```python
from build123d import *

# Parameters (mm, degrees)
SKETCH045_W     = 10
SKETCH045_H     = 80
PAD018_DEPTH    = 7
SKETCH046_R     = 1.4
POCKET026_DEPTH = 8
SKETCH047_R     = 3.5
POCKET027_DEPTH = 80.001


with BuildPart() as part:
    # Sketch045 → Pad018 (new body)
    with BuildSketch(Plane.XY):
        with Locations((100, 0)):
            Rectangle(SKETCH045_W, SKETCH045_H)
    extrude(amount=PAD018_DEPTH)

    # Sketch046 (on Face5 of Pad018) → Pocket026 (cut)
    with BuildSketch(Plane(origin=(0, 0, 0), x_dir=(1, 0, 0), z_dir=(0, 0, -1))):
        with Locations((100, 30)):
            Circle(SKETCH046_R)
        with Locations((100, -30)):
            Circle(SKETCH046_R)
    extrude(amount=-POCKET026_DEPTH, mode=Mode.SUBTRACT)

    # Sketch047 (on Face6 of Pocket026) → Pocket027 (cut, through all)
    with BuildSketch(Plane.XZ.offset(40)):
        with Locations((107.358391, 3.5)):
            Circle(SKETCH047_R)
        with Locations((92.471756, 3.5)):
            Circle(SKETCH047_R)
    extrude(amount=-POCKET027_DEPTH, mode=Mode.SUBTRACT)


with BuildPart() as part_1:
    # Body006 placement: moved
    add(part.part.moved(Location((0, 0, 36.5))))


solid = part_1.part
```
Here's how the part is built. I have some questions about the finished solid (model axes, mm). Round coordinates to 2 decimals unless told otherwise and drop trailing zeros. Order: outer loops, then holes, each group sorted by start corner. A loop starts at its lowest first (then second) coordinate and runs counter-clockwise, first axis right, second up. Notation, with made-up numbers: M 26,83 L 39,83 A8 cw 39,93 Z; hole C 45,57 d3. An arc over 180 degrees is marked long. One line per question, with ' | ' between items.
1) For pin 1 Ø3 at (y, z) = (-24.5, 40.5) entering from -X, with a flat end and sliding along its axis, tell me the tip position at first contact or that it passes through.
Working result:
pin 1: x = 95.34
2) I want a section at B-B, the plane x = 100. Write out the boundary of the cut face in (y, z).
Working result:
outline: M -40,36.5 L -31.4,36.5 L -31.4,43.5 L -40,43.5 Z; M -28.6,36.5 L 28.6,36.5 L 28.6,43.5 L -28.6,43.5 Z; M 31.4,36.5 L 40,36.5 L 40,43.5 L 31.4,43.5 Z
3) I need wall thicknesses on line 1 along Y through (x, z) = (100, 41.75); line 2 along Z through (x, y) = (104.5, 11); line 3 along Y through (x, z) = (99.5, 38). Which ranges of each line are inside material? Lowest first, please.
Working result:
line 1: -40 to -31.4, -28.6 to 28.6, 31.4 to 40 | line 2: 36.5 to 37.98, 42.02 to 43.5 | line 3: -40 to -31.31, -28.69 to 28.69, 31.31 to 40
4) I want a section at D-D, the plane y = 21.5. Write out the boundary of the cut face in (x, z), then the cut area to 3 significant figures.
Working result:
outline: M 95,36.5 L 105,36.5 L 105,37.41 A3.5 cw 105,42.59 L 105,43.5 L 95,43.5 L 95,42.42 A3.5 cw 95,37.58 Z | area: 62.7 mm²
5) I want a section at A-A, the plane y = -30. Write out the boundary of the cut face in (x, z), then the cut area to 3 significant figures.
Working result:
outline: M 95,36.5 L 98.6,36.5 L 98.6,43.5 L 95,43.5 L 95,42.42 A3.5 cw 95,37.58 Z; M 101.4,36.5 L 105,36.5 L 105,37.41 A3.5 cw 105,42.59 L 105,43.5 L 101.4,43.5 Z | area: 43.1 mm²
6) I want a section at C-C, the plane z = 41. Write out the boundary of the cut face in (x, y), then the cut area to 3 significant figures.
Working result:
outline: M 95.83,-40 L 104,-40 L 104,40 L 95.83,40 Z; hole C 100,-30 d2.8; hole C 100,30 d2.8 | area: 642 mm²
7) If we mould it in two halves opening along Y, with no side actions, what happens to faces 1 (the face through (103.86, -0.56, 40.04)), 2 (the face through (98.97, 29.05, 39.95)), 3 (the face through (100, 40, 40))? For each: +Y half, -Y half, draft (parallel to the pull), parting line (faces both ways), or undercut.
Working result:
face 1: draft | face 2: undercut | face 3: +Y half
